Part model, mm, in its own coordinate system. Face numbers are marked on the shaded views. A direction names the side the tool comes from. Round coordinates to 2 decimals unless told otherwise and drop trailing zeros. Order: outer loops, then holes, each group sorted by start corner. A loop starts at its lowest first (then second) coordinate and runs counter-clockwise, first axis right, second up. Notation, with made-up numbers: (50.25, 38.25) - (75.25, 38.25) arc R26 ccw to (75.25, 63.25) - close; hole circle Ø7 at (-2.75, -19). An arc over 180 degrees is marked (long way). Answer as a JSON object with one key per item and string values.
Autodesk Inventor part; units mm, degrees
ref_plane "YZ Plane" through (0, 0, 0) normal (1, 0, 0) x (0, 1, 0)
ref_plane "XZ Plane" through (0, 0, 0) normal (0, 1, 0) x (-1, 0, 0)
ref_plane "XY Plane" through (0, 0, 0) normal (0, 0, 1) x (1, 0, 0)
sketch "Sketch1" plane through (0, 0, 0) normal (0, 0, 1) x (1, 0, 0)
  line L0 (-6, 5) -> (6, 5)
  line L1 (6, 5) -> (6, -5)
  line L2 (6, -5) -> (-6, -5)
  line L3 (-6, -5) -> (-6, 5)
  line L4 (-6, 5) -> (6, -5) construction
  line L5 (6, 5) -> (-6, -5) construction
  point P0 (0, 0)
  dimension "d0" = 12
  dimension "d1" = 10
extrude "Extrusion1" add sketch "Sketch1" along normal blind 24.25
sketch "Sketch2" plane through (0, 0, 24.25) normal (0, 0, 1) x (1, 0, 0)
  circle A0 centre (0, 0) radius 2
  dimension "d4" = 4
extrude "Extrusion2" add sketch "Sketch2" along normal blind 1
sketch "Sketch3" plane through (0, 0, 0) normal (0, 0, -1) x (-1, 0, 0)
  circle A0 centre (0, 0) radius 2
  dimension "d7" = 4
extrude "Extrusion3" add sketch "Sketch3" along normal blind 1
sketch "Sketch4" plane through (0, 0, -1) normal (0, 0, -1) x (-1, 0, 0)
  circle A0 centre (0, 0) radius 1.5
  line L0 (-1.5, 1) -> (1.5, 1)
  line L1 (1.5, 1) -> (1.5, -1.5)
  line L2 (1.5, -1.5) -> (-1.5, -1.5)
  line L3 (-1.5, -1.5) -> (-1.5, 1)
  point P0 (1.118, 1)
  point P1 (-1.118, 1)
  dimension "d10" = 3
  dimension "d11" = 2.5
extrude "Extrusion4" add sketch "Sketch4" along normal blind 4 contours A0 L0 picked at (-0.0419, 0.0796)
fillet "Fillet1" radius 1 8 edges at (6, 5, 12.125) (-6, 5, 12.125) (6, -5, 12.125) (-6, -5, 12.125) (0, 5, 24.25) (6, 0, 24.25) (-6, 0, 24.25) (0, -5, 24.25)
sketch "Sketch5" plane through (0, 0, 0) normal (0, 0, -1) x (-1, 0, 0)
  arc A0 (5, -5) -> (6, -4) centre (5, -4) ccw
  line L0 (6, 4) -> (6, -4)
  arc A1 (6, 4) -> (5, 5) centre (5, 4) ccw
  line L1 (-5, 5) -> (5, 5)
  arc A2 (-5, 5) -> (-6, 4) centre (-5, 4) ccw
  line L2 (-6, -4) -> (-6, 4)
  arc A3 (-6, -4) -> (-5, -5) centre (-5, -4) ccw
  line L3 (5, -5) -> (-5, -5)
  circle A4 centre (0, 0) radius 2
  point P0 (-4.5, 0)
  point P1 (4.5, 0)
  dimension "d15" = 4.5
  dimension "d16" = 4.5
hole "Hole1" at (4.5, 0, 0) at (-4.5, 0, 0) direction (0, 0, 1) diameter 1.221 depth 1
properties part number "1800rpm Brushed Motor"
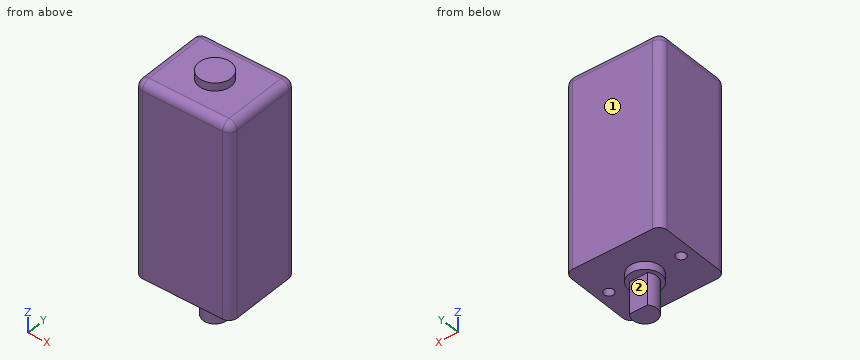
Item 1: Cut at D-D (y = -3.5). Write the cut outline in (x, z), plus the area to 3 significant figures.
Taken from the geometry:
{"outline": "(-6, 0) - (6, 0) - (6, 23.25) arc R1 ccw to (5, 24.25) - (-5, 24.25) arc R1 ccw to (-6, 23.25) - close", "area": "291 mm2"}
Item 2: Cut at A-A (x = 0). Write the cut outline in (y, z).
Taken from the geometry:
{"outline": "(-5, 0) - (-2, 0) - (-2, -1) - (-1.5, -1) - (-1.5, -5) - (1, -5) - (1, -1) - (2, -1) - (2, 0) - (5, 0) - (5, 23.25) arc R1 ccw to (4, 24.25) - (2, 24.25) - (2, 25.25) - (-2, 25.25) - (-2, 24.25) - (-4, 24.25) arc R1 ccw to (-5, 23.25) - close"}
Item 3: Probe L1, parallel to X at y = 0, z = 0.45; L2, parallel to Y at x = 4.5, z = 0.6; L3, parallel to Z at x = 2.75, y = 1.5. List the from-to ranges inside material, lowest first. Write a range as from..to.
Taken from the geometry:
{"L1": "-6..-5.11, -3.89..3.89, 5.11..6", "L2": "-5..-0.61, 0.61..5", "L3": "0..24.25"}
Item 4: Cut at B-B (y = 0). Write the cut outline in (x, z), plus the area to 3 significant figures.
Taken from the geometry:
{"outline": "(-6, 0) - (-5.11, 0) - (-5.11, 1) - (-3.89, 1) - (-3.89, 0) - (-2, 0) - (-2, -1) - (-1.5, -1) - (-1.5, -5) - (1.5, -5) - (1.5, -1) - (2, -1) - (2, 0) - (3.89, 0) - (3.89, 1) - (5.11, 1) - (5.11, 0) - (6, 0) - (6, 23.25) arc R1 ccw to (5, 24.25) - (2, 24.25) - (2, 25.25) - (-2, 25.25) - (-2, 24.25) - (-5, 24.25) arc R1 ccw to (-6, 23.25) - close", "area": "308 mm2"}
Item 5: Drop flat-ended pins along their axis: P1, Ø5, axis at x = 3.5, y = 1, coming from the -Z side; P2, Ø1, axis at x = 4.5, y = 0, coming from the +Z side; P3, Ø1.8, axis at x = 0.5, z = -3.5, coming from the +Y side. Give the stop position or say it passes through.
Taken from the geometry:
{"P1": "z = -5", "P2": "z = 24.25", "P3": "y = 1"}
Item 6: Tool access for the marked faces 1 and 2: list every direction of +Z, -Z, +X, -X, +Y, -Y with a clear straight run to the whole face (end or side of a thin tool).
Taken from the geometry:
{"face 1": "+Z, -Z, +X, -X, +Y", "face 2": "-Z, +X, -X, +Y"}
Item 7: Cut at C-C (x = 4.5). Write the cut outline in (y, z).
Taken from the geometry:
{"outline": "(-5, 0) - (-0.61, 0) - (-0.61, 1) - (0.61, 1) - (0.61, 0) - (5, 0) - (5, 23.25) arc R1 ccw to (4, 24.25) - (-4, 24.25) arc R1 ccw to (-5, 23.25) - close"}
